Check sheet for the modelled part. Datum: model origin and axes. Units: mm. A direction names the side the tool comes from. Coordinates: 2 decimals unless noted, no trailing zeros. Loops run counter-clockwise (first coordinate to the right, second up) from the corner with the lowest first, then second, coordinate; pieces in that order, holes last.
from build123d import *

# Parameters (mm, degrees)
CROQUIS1_W              = 50
CROQUIS1_H              = 8
CROQUIS1_R              = 1.932766006
CROQUIS1_R_2            = 0.996557478
SALIENTE_EXTRUIR1_DEPTH = 4
CROQUIS2_W              = 13
CROQUIS2_H              = 1.180512064
CORTAR_EXTRUIR1_DEPTH   = 27.551836095


with BuildPart() as part:
    # Croquis1 → Saliente-Extruir1 (new, symmetric)
    with BuildSketch(Plane.XY):
        Rectangle(CROQUIS1_W, CROQUIS1_H)
        with Locations((-21.377815108, 0)):
            Circle(CROQUIS1_R, mode=Mode.SUBTRACT)
        with Locations((22, 0)):
            Circle(CROQUIS1_R_2, mode=Mode.SUBTRACT)
    extrude(amount=SALIENTE_EXTRUIR1_DEPTH, both=True)

    # Croquis2 → Cortar-Extruir1 (cut, through all)
    with BuildSketch(Plane(origin=(0, 4, 0), x_dir=(1, 0, 0), z_dir=(0, 1, 0))):
        with Locations((25, 0)):
            Rectangle(CROQUIS2_W, CROQUIS2_H)
    extrude(amount=-CORTAR_EXTRUIR1_DEPTH, mode=Mode.SUBTRACT)


solid = part.part
(1) Set-up check for faces 4 (the face through (-23.31, 0.08, -0.06)), 5 (the face through (21, 1, 0.59)): record each of +Z, -Z, +X, -X, +Y, -Y from which the full face is reachable in a straight line by a thin tool's end or side.
(2) Draft check along Z on faces 1 (the face through (22.92, -0.38, -2.32)), 2 (the face through (0, 0, 4)), 3 (the face through (21, 1, -0.59)). Enter one of: pulls with the +Z half, pulls with the -Z half, needs draft (parallel to the pull), parting line crosses it, or undercut.
(3) Scan lines: line 1 along Y through (x, z) = (22, -2.1); line 2 along X through (y, z) = (-0.5, 2); line 3 along X through (y, z) = (0.25, 1.75). Record each from-to range of solid material in increasing order.
(4) Section check D-D, the plane x = -20. Enter the section's corners in (y, z).
(5) Gauge pin test, flat ends, axial feed: P1, Ø2.5, axis at x = 22, y = 0, coming from the -Z side; P2, Ø0.6, axis at y = -2, z = 0, coming from the +X side. Record the tip position at first contact, or that the pin passes through.
(6) Section check A-A, the plane y = 0. Enter the section's corners in (x, z), plus the area to 3 significant figures.
(7) Section check C-C, the plane y = -2.5. Enter the section's corners in (x, z).
(8) Section check B-B, the plane x = 22. Enter the section's corners in (y, z), plus the area to 3 significant figures.
Determined:
1. face 4: +Z, -Z
1. face 5: +X, +Y, -Y
2. face 1: needs draft
2. face 2: pulls with the +Z half
2. face 3: undercut
3. line 1: y = -4 to -1, 1 to 4
3. line 2: x = -25 to -23.24, -19.51 to 21.14, 22.86 to 25
3. line 3: x = -25 to -23.29, -19.46 to 21.04, 22.96 to 25
4. outline: (-4, -4) - (-1.36, -4) - (-1.36, 4) - (-4, 4) - close; (1.36, -4) - (4, -4) - (4, 4) - (1.36, 4) - close
5. P1: stops at z = -4
5. P2: stops at x = 18.5
6. outline: (-25, -4) - (-23.31, -4) - (-23.31, 4) - (-25, 4) - close; (-19.45, -4) - (21, -4) - (21, -0.59) - (18.5, -0.59) - (18.5, 0.59) - (21, 0.59) - (21, 4) - (-19.45, 4) - close; (23, -4) - (25, -4) - (25, -0.59) - (23, -0.59) - close; (23, 0.59) - (25, 0.59) - (25, 4) - (23, 4) - close
6. area: 348 mm2
7. outline: (-25, -4) - (25, -4) - (25, -0.59) - (18.5, -0.59) - (18.5, 0.59) - (25, 0.59) - (25, 4) - (-25, 4) - close
8. outline: (-4, -4) - (-1, -4) - (-1, -0.59) - (-4, -0.59) - close; (-4, 0.59) - (-1, 0.59) - (-1, 4) - (-4, 4) - close; (1, -4) - (4, -4) - (4, -0.59) - (1, -0.59) - close; (1, 0.59) - (4, 0.59) - (4, 4) - (1, 4) - close
8. area: 41.0 mm2
